The model under review builds one solid part; all positions refer to its coordinate system, in mm. A direction names the side the tool comes from. Give positions to 0.01 mm unless a question says otherwise; leave off trailing zeros. Order: outer loops, then holes, each group sorted by start corner. A loop starts at its lowest first (then second) coordinate and runs counter-clockwise, first axis right, second up. Notation, with made-up numbers: (-17.75, -24.5) -> (5.25, -24.5) arc R19 cw to (5.25, -14.5) -> close; hole circle Ø3 at (-33, 68.5). An arc over 180 degrees is marked (long way). Use one line per item in the form item = value.
```python
from build123d import *

# Parameters (mm, degrees)
SKETCH1_W           = 26
SKETCH1_H           = 52
BOSS_EXTRUDE1_DEPTH = 30
SKETCH2_W           = 1.5
SKETCH2_H           = 27
CUT_EXTRUDE1_DEPTH  = 53
SKETCH3_OUTSIDE_W   = 41.084
SKETCH3_OUTSIDE_H   = 67.084
SKETCH3_OUTSIDE_W_2 = 17
SKETCH3_OUTSIDE_H_2 = 17
SKETCH3_OUTSIDE_H_3 = 11.7
SKETCH3_OUTSIDE_W_3 = 3
SKETCH3_OUTSIDE_H_4 = 20.15
CUT_EXTRUDE2_DEPTH  = 27
SKETCH4_W           = 17
SKETCH4_H           = 11.7
CUT_EXTRUDE3_DEPTH  = 17
SKETCH5_R           = 2.15
CUT_EXTRUDE4_DEPTH  = 27


with BuildPart() as part:
    # Sketch1 → Boss-Extrude1 (new body)
    with BuildSketch(Plane(origin=(0, 0, 0), x_dir=(1, 0, 0), z_dir=(0, 1, 0))):
        with Locations((13, 26)):
            Rectangle(SKETCH1_W, SKETCH1_H)
    extrude(amount=BOSS_EXTRUDE1_DEPTH)

    # Sketch2 → Cut-Extrude1 (cut, through all)
    with BuildSketch(Plane(origin=(0, 0, -52), x_dir=(-1, 0, 0), z_dir=(0, 0, -1))):
        with Locations((-22.25, 16.5)):
            Rectangle(SKETCH2_W, SKETCH2_H)
        with Locations((-3.75, 16.5)):
            Rectangle(SKETCH2_W, SKETCH2_H)
    extrude(amount=-CUT_EXTRUDE1_DEPTH, mode=Mode.SUBTRACT)

    # Sketch3 outside → Cut-Extrude2 (cut)
    with BuildSketch(Plane(origin=(0, 30, 0), x_dir=(1, 0, 0), z_dir=(0, 1, 0))):
        with Locations((13, 26)):
            Rectangle(SKETCH3_OUTSIDE_W, SKETCH3_OUTSIDE_H)
        with Locations((13, 41.95)):
            Rectangle(SKETCH3_OUTSIDE_W_2, SKETCH3_OUTSIDE_H_2, mode=Mode.SUBTRACT)
        with Locations((13, 26)):
            Rectangle(SKETCH3_OUTSIDE_W_2, SKETCH3_OUTSIDE_H_3, mode=Mode.SUBTRACT)
        with Locations((13, 10.05)):
            Rectangle(SKETCH3_OUTSIDE_W_2, SKETCH3_OUTSIDE_H_2, mode=Mode.SUBTRACT)
        with Locations((1.5, 41.925)):
            Rectangle(SKETCH3_OUTSIDE_W_3, SKETCH3_OUTSIDE_H_4, mode=Mode.SUBTRACT)
        with Locations((24.5, 41.925)):
            Rectangle(SKETCH3_OUTSIDE_W_3, SKETCH3_OUTSIDE_H_4, mode=Mode.SUBTRACT)
        with Locations((1.5, 10.075)):
            Rectangle(SKETCH3_OUTSIDE_W_3, SKETCH3_OUTSIDE_H_4, mode=Mode.SUBTRACT)
        with Locations((24.5, 10.075)):
            Rectangle(SKETCH3_OUTSIDE_W_3, SKETCH3_OUTSIDE_H_4, mode=Mode.SUBTRACT)
    extrude(amount=-CUT_EXTRUDE2_DEPTH, mode=Mode.SUBTRACT)

    # Sketch4 → Cut-Extrude3 (cut)
    with BuildSketch(Plane(origin=(0, 30, 0), x_dir=(1, 0, 0), z_dir=(0, 1, 0))):
        with Locations((13, 26)):
            Rectangle(SKETCH4_W, SKETCH4_H)
    extrude(amount=-CUT_EXTRUDE3_DEPTH, mode=Mode.SUBTRACT)

    # Sketch5 → Cut-Extrude4 (cut, through all)
    with BuildSketch(Plane.ZY):
        with Locations((-42, 25)):
            Circle(SKETCH5_R)
        with Locations((-42, 10)):
            Circle(SKETCH5_R)
        with Locations((-10, 25)):
            Circle(SKETCH5_R)
        with Locations((-10, 10)):
            Circle(SKETCH5_R)
    extrude(amount=-CUT_EXTRUDE4_DEPTH, mode=Mode.SUBTRACT)


solid = part.part
```
1. Add section D-D on y = 25. Count the separate pieces of the cut face and the enclosed holes in it, then the cut area to 3 significant figures.
Values:
separate_pieces = 12
enclosed_holes = 0
area = 622 mm^2
2. Add section C-C on z = -35. Give the boundary of the cut face in (x, y), then the cut area to 3 significant figures.
Values:
outline = (0, 0) -> (26, 0) -> (26, 30) -> (23, 30) -> (23, 3) -> (21.5, 3) -> (21.5, 30) -> (4.5, 30) -> (4.5, 3) -> (3, 3) -> (3, 30) -> (0, 30) -> close
area = 699 mm^2
3. For pin 1 Ø5 at (x, y) = (18, 6.5) entering from -Z; pin 2 Ø3 at (y, z) = (12, -10.5) entering from -X; pin 3 Ø12 at (x, y) = (11.5, 23.5) entering from +Z, all flat-tipped, find the tip position at first contact; note any pin that passes through.
Values:
pin_1 = -50.45
pin_2 = 0
pin_3 = -1.55
4. The part is to be moulded in two halves that separate along Z. For faces 4 (the face through (12, 2.7, 0)), 5 (the face through (24.479, 24.177, -40.014)), 6 (the face through (23, 16, -10)), say which applies: +Z half, -Z half, draft (parallel to the pull), parting line (faces both ways), or undercut.
Values:
face_4 = +Z half
face_5 = undercut
face_6 = draft
5. Add section B-B on x = 13.5. Give the boundary of the cut face in (y, z).
Values:
outline = (0, -52) -> (3, -52) -> (3, -50.45) -> (30, -50.45) -> (30, -33.45) -> (3, -33.45) -> (3, -31.85) -> (13, -31.85) -> (13, -20.15) -> (3, -20.15) -> (3, -18.55) -> (30, -18.55) -> (30, -1.55) -> (3, -1.55) -> (3, 0) -> (0, 0) -> close; hole circle Ø4.3 at (10, -42); hole circle Ø4.3 at (10, -10); hole circle Ø4.3 at (25, -42); hole circle Ø4.3 at (25, -10)
6. For L1, parallel to Y at x = 16.5, z = -10; L2, parallel to X at y = 25.75, z = -14; L3, parallel to Z at x = 5.75, y = 6, list the stretches that pass through material, from the lowest coordinate up.
Values:
L1 = 0 to 7.85, 12.15 to 22.85, 27.15 to 30
L2 = 0 to 3, 4.5 to 21.5, 23 to 26
L3 = -50.45 to -33.45, -31.85 to -20.15, -18.55 to -1.55
7. Add section A-A on y = 17.5. Give the boundary of the cut face in (x, z), then the cut area to 3 significant figures.
Values:
outline = (0, -52) -> (3, -52) -> (3, -31.85) -> (0, -31.85) -> close; (0, -20.15) -> (3, -20.15) -> (3, 0) -> (0, 0) -> close; (4.5, -50.45) -> (21.5, -50.45) -> (21.5, -33.45) -> (4.5, -33.45) -> close; (4.5, -18.55) -> (21.5, -18.55) -> (21.5, -1.55) -> (4.5, -1.55) -> close; (23, -52) -> (26, -52) -> (26, -31.85) -> (23, -31.85) -> close; (23, -20.15) -> (26, -20.15) -> (26, 0) -> (23, 0) -> close
area = 820 mm^2
8. Tool access review of faces 1 (the face through (1, 17, -31.85)), 2 (the face through (24, 17, -31.85)), 3 (the face through (13, 8, -20.15)): name each direction out of +Z, -Z, +X, -X, +Y, -Y from which nothing blocks a thin tool from reaching the whole face with its end or side.
Values:
face_1 = -X, +Y
face_2 = +X, +Y
face_3 = +Y
